Source: CAD feature listing. Evaluate the final solid. Frame: model axes, mm. A direction names the side the tool comes from. Coordinates: 2 decimals unless noted, no trailing zeros. Write each loop counter-clockwise with the first axis right and the second up, starting at its lowest first coordinate (ties: lowest second). Pieces come first, ordered by that corner, then holes. Notation, with made-up numbers: M 55.25,67 L 62.25,67 A29 ccw 62.25,89 Z; hole C 0,86.5 d5. An arc over 180 degrees is marked long. Write item = value, one per line. Start each with the question number.
1. Section query A-A (y = 0). Output: boundary loops of the cut face in (x, z).
2. Line query: line 1 along X through (y, z) = (0, -256.9); line 2 along Y through (x, z) = (0, 114). Output: solid intervals per line, ascending.
3. Pin query (flat end, axial travel): pin 1 Ø10 at (y, z) = (-12, 90) entering from -X; pin 2 Ø10 at (x, z) = (8, -3) entering from -Y; pin 3 Ø14.5 at (x, y) = (0, 0) entering from -Z; pin 4 Ø3 at (x, z) = (-11.5, -178.5) entering from +Y. Return the tip coordinate at first contact, or that it passes through.
4. Pull-direction query (X, two-part tool) for faces 1 (the face through (-14.985, 0.66, 3.332)), 2 (the face through (9, 9, 258)), 3 (the face through (14.5, -3.22, -248.73)); classes: pulls with the +X half, pulls with the -X half, needs draft (parallel to the pull), parting line crosses it, or undercut.
5. Access query for faces 4 (the face through (-5.362, 12.932, -255.028)), 5 (the face through (3.86, 12.26, 248.73)), 6 (the face through (5.362, 12.932, 255.028)). Directions: +Z, -Z, +X, -X, +Y, -Y. A direction counts if a zero-diameter tool reaches every point of the face in a straight line with its end or side. Return the directions, or none.
6. Section query C-C (z = 38.5). Output: boundary loops of the cut face in (x, y), then the cut area to 3 significant figures.
Autodesk Inventor part; units mm, degrees
ref_plane "YZ Plane" through (0, 0, 0) normal (1, 0, 0) x (0, 1, 0)
ref_plane "XZ Plane" through (0, 0, 0) normal (0, 1, 0) x (-1, 0, 0)
ref_plane "XY Plane" through (0, 0, 0) normal (0, 0, 1) x (1, 0, 0)
sketch "Sketch1" plane through (0, 0, 0) normal (0, 0, 1) x (1, 0, 0)
  circle A0 centre (0, 0) radius 15
  circle A1 centre (0, 0) radius 17
  dimension "d0" = 30
  dimension "d1" = 2
extrude "Extrusion1" add sketch "Sketch1" against normal mid plane 476
sketch "Sketch2" plane through (0, 0, 0) normal (1, 0, 0) x (0, 1, 0)
  line L0 (15, -238) -> (15, 238)
  line L1 (17, 238) -> (17, -238)
  line L2 (14, 253) -> (14, 258)
  line L3 (14, 258) -> (12, 258)
  line L4 (12, 258) -> (12, 253)
  line L5 (17, 238) -> (-17, 238)
  line L6 (14, 253) -> (17, 238)
  line L7 (12, 253) -> (15, 238)
  line L8 (0, 0) -> (0, 22.4237)
  dimension "d4" = 2
  dimension "d5" = 2
  dimension "d8" = 12
  dimension "d10" = 5
  dimension "d13" = 20
revolve "Revolution1" add sketch "Sketch2" angle 360 about axis through (0, 0, 0) along (0, 0, 1)
fillet "Fillet2" radius 1 1 edges at (0, -14, 258)
mirror "Mirror1" about plane through (0, 0, 0) normal (0, 0, 1) of "Revolution1", "Fillet2"
equation "\"d5\" = d4"
properties part number "OuterGlassTube" material "Glass"
Results are:
q1.outline = M -17,-238 L -14,-253 L -14,-257 A1 ccw -13,-258 L -12,-258 L -12,-253 L -15,-238 L -15,238 L -12,253 L -12,258 L -13,258 A1 ccw -14,257 L -14,253 L -17,238 Z; M 12,-258 L 13,-258 A1 ccw 14,-257 L 14,-253 L 17,-238 L 17,238 L 14,253 L 14,257 A1 ccw 13,258 L 12,258 L 12,253 L 15,238 L 15,-238 L 12,-253 Z
q2.line_1 = -14 to -12, 12 to 14
q2.line_2 = -17 to -15, 15 to 17
q3.pin_1 = -15.49
q3.pin_2 = -16.73
q3.pin_3 = through
q3.pin_4 = 13.75
q4.face_1 = undercut
q4.face_2 = needs draft
q4.face_3 = parting line crosses it
q5.face_4 = -Z
q5.face_5 = none
q5.face_6 = +Z
q6.outline = C 0,0 d34; hole C 0,0 d30
q6.area = 201 mm^2
